```python
from build123d import *

# Parameters (mm, degrees)
BOSS_EXTRUDE1_DEPTH     = 3.175
SKETCH3_R               = 2.54
CUT_EXTRUDE4_DEPTH      = 4.175
CUT_EXTRUDE4_DEPTH_BACK = 1


with BuildPart() as part:
    # Sketch2 → Boss-Extrude1 (new body)
    with BuildSketch(Plane.XY):
        Polygon((-79.260302653, 74.809862941), (-93.829144137, 54.003401016), (-30.387651704, 9.581189779), (0, 0), (73.861366343, 0), (73.861366343, 25.4), (0, 128.712625375), (-25.4, 128.712625375), align=None)
        with BuildLine():
            Line((-59.82155239, 74.809862941), (-30.48, 74.809862941))
            ThreePointArc((-30.48, 74.809862941), (-26.887897552, 76.297760492), (-25.4, 79.889862941))
            Line((-25.4, 79.889862941), (-25.4, 109.254546205))
            ThreePointArc((-25.4, 109.254546205), (-28.536892808, 113.948237124), (-34.073517496, 112.845233049))
            Line((-34.073517496, 112.845233049), (-63.415069886, 83.480549784))
            ThreePointArc((-63.415069886, 83.480549784), (-64.51447734, 77.944906536), (-59.82155239, 74.809862941))
        make_face(mode=Mode.SUBTRACT)
        with BuildLine():
            Line((-55.893609183, 69.729862941), (-30.48, 69.729862941))
            ThreePointArc((-30.48, 69.729862941), (-26.887897552, 68.241965389), (-25.4, 64.649862941))
            Line((-25.4, 64.649862941), (-25.4, 46.855062218))
            ThreePointArc((-25.4, 46.855062218), (-28.134317045, 42.349047185), (-33.393768297, 42.693769833))
            Line((-33.393768297, 42.693769833), (-58.80737748, 60.488570556))
            ThreePointArc((-58.80737748, 60.488570556), (-60.738491293, 66.177448402), (-55.893609183, 69.729862941))
        make_face(mode=Mode.SUBTRACT)
        with BuildLine():
            Line((7.797059491, 36.347810077), (39.049758479, 56.13093342))
            ThreePointArc((39.049758479, 56.13093342), (41.318484722, 59.449422894), (40.465204003, 63.377705364))
            Line((40.465204003, 63.377705364), (9.212505015, 107.092011536))
            ThreePointArc((9.212505015, 107.092011536), (3.528665973, 108.974887007), (0, 104.137556882))
            Line((0, 104.137556882), (0, 40.640127367))
            ThreePointArc((0, 40.640127367), (2.630128801, 36.189899159), (7.797059491, 36.347810077))
        make_face(mode=Mode.SUBTRACT)
        with BuildLine():
            Line((14.80606505, 34.772317291), (42.476873448, 52.288084993))
            ThreePointArc((42.476873448, 52.288084993), (46.177688514, 52.979604073), (49.338173329, 50.93373836))
            Line((49.338173329, 50.93373836), (61.755602511, 33.417970658))
            ThreePointArc((61.755602511, 33.417970658), (62.124193324, 28.147457497), (57.61136212, 25.4))
            Line((57.61136212, 25.4), (17.52312454, 25.4))
            ThreePointArc((17.52312454, 25.4), (12.644017458, 29.065533994), (14.80606505, 34.772317291))
        make_face(mode=Mode.SUBTRACT)
    extrude(amount=BOSS_EXTRUDE1_DEPTH)

    # Sketch3 → Cut-Extrude4 (cut, two sides)
    with BuildSketch(Plane.XY) as cut_extrude4_sk:
        with Locations((-12.7, 57.15)):
            Circle(SKETCH3_R)
        with Locations((6.35, 12.7)):
            Circle(SKETCH3_R)
        with Locations((-28.304846444, 23.626631112)):
            Circle(SKETCH3_R)
        with Locations((-38.708077406, 30.911051854)):
            Circle(SKETCH3_R)
        with Locations((-49.111308369, 38.195472596)):
            Circle(SKETCH3_R)
        with Locations((-59.514539331, 45.479893337)):
            Circle(SKETCH3_R)
        with Locations((-69.917770294, 52.764314079)):
            Circle(SKETCH3_R)
        with Locations((-80.321001256, 60.048734821)):
            Circle(SKETCH3_R)
        with Locations((-12.7, 69.85)):
            Circle(SKETCH3_R)
        with Locations((-12.7, 82.55)):
            Circle(SKETCH3_R)
        with Locations((-12.7, 95.25)):
            Circle(SKETCH3_R)
        with Locations((-12.7, 107.95)):
            Circle(SKETCH3_R)
        with Locations((-12.7, 120.65)):
            Circle(SKETCH3_R)
        with Locations((19.05, 12.7)):
            Circle(SKETCH3_R)
        with Locations((31.75, 12.7)):
            Circle(SKETCH3_R)
        with Locations((44.45, 12.7)):
            Circle(SKETCH3_R)
        with Locations((57.15, 12.7)):
            Circle(SKETCH3_R)
        with Locations((69.85, 12.7)):
            Circle(SKETCH3_R)
    extrude(amount=CUT_EXTRUDE4_DEPTH, mode=Mode.SUBTRACT)
    extrude(cut_extrude4_sk.sketch, amount=-CUT_EXTRUDE4_DEPTH_BACK, mode=Mode.SUBTRACT)


solid = part.part
```
Model file for the job. Use its own axes, mm. A direction names the side the tool comes from. Give positions to 0.01 mm unless a question says otherwise; leave off trailing zeros. Loops run counter-clockwise (first coordinate to the right, second up) from the corner with the lowest first, then second, coordinate; pieces in that order, holes last. Notation, with made-up numbers: (81.5, -1.75) -> (100.5, -1.75) arc R11 cw to (100.5, 10.25) -> close; hole circle Ø7 at (29.5, 52). An arc over 180 degrees is marked (long way). Use CSV: the item, a comma, the result in double quotes. Start each with the question number.
1) Flat gauge pins, fed straight in: pin 1 Ø6 at (x, y) = (-12.7, 107.95) entering from +Z (3 decimals); pin 2 Ø1.5 at (x, z) = (-38, 1) entering from -Y; pin 3 Ø1 at (x, z) = (-50.5, 2) entering from +Y; pin 4 Ø1 at (y, z) = (71, 1) entering from +X. Where does each tip first touch, or does it go through?
2) Tool access for faces 1 (the flat face through (-86.443, 64.552, 1.565)), 2 (the flat face through (23.2, 46.1, 1.6)): list every direction of +Z, -Z, +X, -X, +Y, -Y with a clear straight run to the whole face (end or side of a thin tool).
3) Slice it at D-D on x = -38.5. Give the cut face in (y, z) (3 decimals).
4) Slice it at B-B on x = -12.7. Give the cut face in (y, z) (3 decimals).
5) Wall check: line 1 (Y direction, x = 22, z = 1.9); line 2 (Y direction, x = -43.5, z = 0.9); line 3 (X direction, y = 39.5, z = 0.25). Give the ranges that are in metal, low to high.
6) Mould opens along Y. For faces 3 (the flat face through (-51.95, 102.14, 1.57)), 4 (the flat face through (36, 0, 2)), 5 (the flat face through (-43, 69.73, 2)) say: released by +Y, released by -Y, zero draft, split by the parting line, or undercut.
7) Slice it at A-A on y = 12.7. Give the cut face in (x, z) (3 decimals), plus the area to 3 significant figures.
8) Slice it at C-C on y = 120.65. Give the cut face in (x, z) (3 decimals).
Computed values:
1,pin 1,"stops at z = 3.175"
1,pin 2,"stops at y = 14.39"
1,pin 3,"stops at y = 104.09"
1,pin 4,"stops at x = 41.62"
2,face 1,"+Z, -Z, -X, +Y"
2,face 2,"+Z, -Z"
3,outline,"(15.262, 0) -> (28.38, 0) -> (28.38, 3.175) -> (15.262, 3.175) -> close; (33.443, 0) -> (46.269, 0) -> (46.269, 3.175) -> (33.443, 3.175) -> close; (69.73, 0) -> (74.81, 0) -> (74.81, 3.175) -> (69.73, 3.175) -> close; (108.415, 0) -> (115.602, 0) -> (115.602, 3.175) -> (108.415, 3.175) -> close"
4,outline,"(4.004, 0) -> (54.61, 0) -> (54.61, 3.175) -> (4.004, 3.175) -> close; (59.69, 0) -> (67.31, 0) -> (67.31, 3.175) -> (59.69, 3.175) -> close; (72.39, 0) -> (80.01, 0) -> (80.01, 3.175) -> (72.39, 3.175) -> close; (85.09, 0) -> (92.71, 0) -> (92.71, 3.175) -> (85.09, 3.175) -> close; (97.79, 0) -> (105.41, 0) -> (105.41, 3.175) -> (97.79, 3.175) -> close; (110.49, 0) -> (118.11, 0) -> (118.11, 3.175) -> (110.49, 3.175) -> close; (123.19, 0) -> (128.713, 0) -> (128.713, 3.175) -> (123.19, 3.175) -> close"
5,line 1,"y = 0 to 25.4, 39.33 to 45.34, 89.21 to 97.94"
5,line 2,"y = 18.76 to 49.77, 69.73 to 74.81, 103.41 to 110.6"
5,line 3,"x = -73.12 to -51.29, -46.93 to 0.13, 12.78 to 22.27, 57.44 to 63.78"
6,face 3,"released by +Y"
6,face 4,"released by -Y"
6,face 5,"undercut"
7,outline,"(-34.842, 0) -> (3.81, 0) -> (3.81, 3.175) -> (-34.842, 3.175) -> close; (8.89, 0) -> (16.51, 0) -> (16.51, 3.175) -> (8.89, 3.175) -> close; (21.59, 0) -> (29.21, 0) -> (29.21, 3.175) -> (21.59, 3.175) -> close; (34.29, 0) -> (41.91, 0) -> (41.91, 3.175) -> (34.29, 3.175) -> close; (46.99, 0) -> (54.61, 0) -> (54.61, 3.175) -> (46.99, 3.175) -> close; (59.69, 0) -> (67.31, 0) -> (67.31, 3.175) -> (59.69, 3.175) -> close; (72.39, 0) -> (73.861, 0) -> (73.861, 3.175) -> (72.39, 3.175) -> close"
7,area,"248 mm^2"
8,outline,"(-33.456, 0) -> (-15.24, 0) -> (-15.24, 3.175) -> (-33.456, 3.175) -> close; (-10.16, 0) -> (5.764, 0) -> (5.764, 3.175) -> (-10.16, 3.175) -> close"
